Input: dimensioned drawing with shaded views. Units: mm. Origin: part minimum x, y, z. Round coordinates to 2 decimals unless told otherwise and drop trailing zeros. Loops run counter-clockwise (first coordinate to the right, second up) from the corner with the lowest first, then second, coordinate; pieces in that order, holes last.
1) Section D-D, the plane z = 4.4. Return loops of the section in (x, y).
2) Draft query along Y for the marked faces 1, 2 and 3. Return one class per face: pulls with the +Y half, pulls with the -Y half, needs draft (parallel to the pull), parting line crosses it, or undercut.
3) Section C-C, the plane x = 63.5. Return loops of the section in (y, z), and give its area (3 significant figures).
4) Section A-A, the plane y = 39.5. Return loops of the section in (x, z), and give its area (3 significant figures).
5) First-contact query: pin 1 (2 mm diameter, centred on y = 9.5, z = 4.5, fed in from +X). Flat tip, straight axial feed; report the tip coordinate or a pass-through.
6) Ray query, line 1 along Y through (x, z) = (39.5, 1.3); line 2 along Y through (x, z) = (58.5, 4.25); line 3 along X through (y, z) = (25.5, 2.6). Return the intervals inside material, ascending.
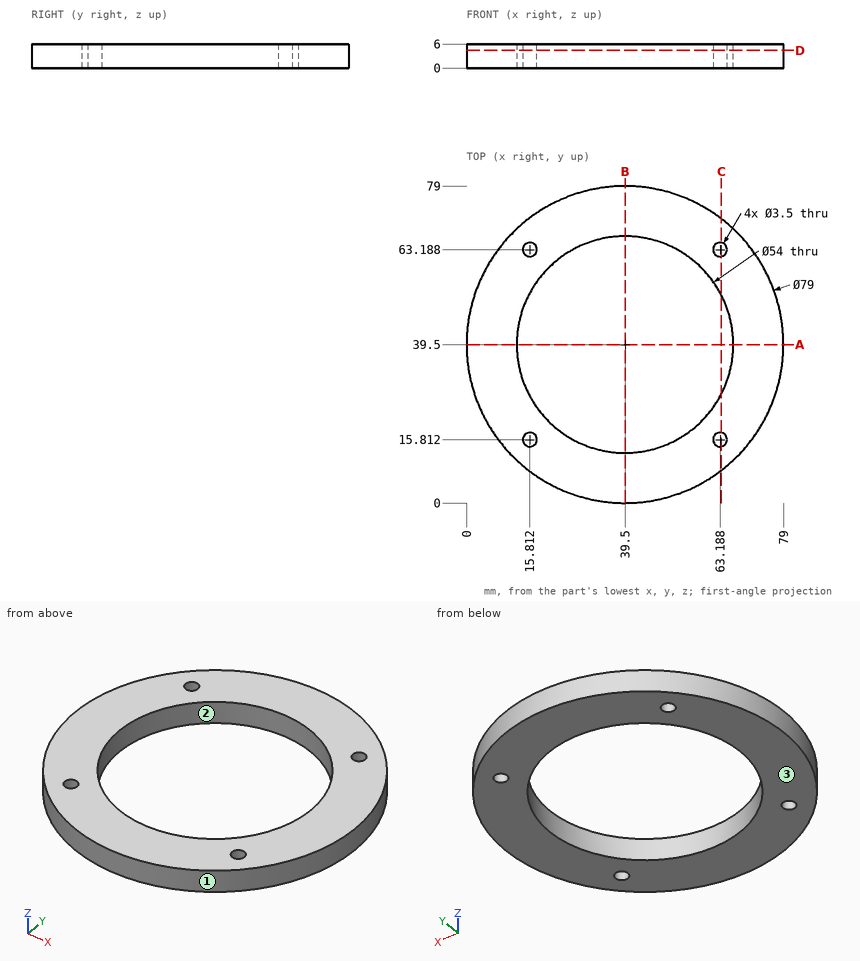
Final values:
1. outline: circle Ø79 at (39.5, 39.5); hole circle Ø54 at (39.5, 39.5); hole circle Ø3.5 at (15.81, 15.81); hole circle Ø3.5 at (15.81, 63.19); hole circle Ø3.5 at (63.19, 15.81); hole circle Ø3.5 at (63.19, 63.19)
2. face 1: parting line crosses it
2. face 2: undercut
2. face 3: needs draft
3. outline: (8.13, 0) - (14.09, 0) - (14.09, 6) - (8.13, 6) - close; (17.53, 0) - (27.13, 0) - (27.13, 6) - (17.53, 6) - close; (51.87, 0) - (61.47, 0) - (61.47, 6) - (51.87, 6) - close; (64.91, 0) - (70.87, 0) - (70.87, 6) - (64.91, 6) - close
3. area: 187 mm2
4. outline: (0, 0) - (12.5, 0) - (12.5, 6) - (0, 6) - close; (66.5, 0) - (79, 0) - (79, 6) - (66.5, 6) - close
4. area: 150 mm2
5. pin 1: stops at x = 66.32
6. line 1: y = 0 to 12.5, 66.5 to 79
6. line 2: y = 4.87 to 20.32, 58.68 to 74.13
6. line 3: x = 2.56 to 16.41, 62.59 to 76.44
